The listing builds one solid part. Answer for the finished solid, in the listing's coordinates (mm). A direction names the side the tool comes from. Give positions to 0.01 mm unless a question says otherwise; leave off trailing zeros. Write each loop counter-clockwise with the first axis right and the second up, starting at its lowest first coordinate (ties: lowest second). Pieces come first, ordered by that corner, then holes.
```python
from build123d import *

# Parameters (mm, degrees)
SKETCH_1_R               = 30.6
EXTRUDE_1_DEPTH          = 24
SKETCH_3_R               = 30.6
EXTRUDE_2_DEPTH          = 0.9
EXTRUDE_2_TAPER          = 73
SKETCH_4_R               = 25.656232643
EXTRUDE_3_DEPTH          = 0.6
SKETCH_5_W               = 51
SKETCH_5_H               = 12
CUT_EXTRUDE_1_DEPTH      = 31.6000001
CUT_EXTRUDE_1_DEPTH_BACK = 31.6000001
SKETCH_6_R               = 2.65
EXTRUDE_4_DEPTH          = 13


with BuildPart() as part:
    # 草图1 → 凸台-拉伸1 (new body)
    with BuildSketch(Plane(origin=(0, 0, 0), x_dir=(1, 0, 0), z_dir=(0, 1, 0))):
        Circle(SKETCH_1_R)
    extrude(amount=EXTRUDE_1_DEPTH)

    # 草图3 → 凸台-拉伸2 (add)
    with BuildSketch(Plane(origin=(0, 24, 0), x_dir=(1, 0, 0), z_dir=(0, 1, 0))):
        Circle(SKETCH_3_R)
    extrude(amount=EXTRUDE_2_DEPTH, taper=EXTRUDE_2_TAPER)

    # 草图4 → 凸台-拉伸3 (add)
    with BuildSketch(Plane(origin=(0, 24.9, 0), x_dir=(1, 0, 0), z_dir=(0, 1, 0))):
        Circle(SKETCH_4_R)
    extrude(amount=EXTRUDE_3_DEPTH)

    # 草图5 → 切除-拉伸1 (cut, two sides)
    with BuildSketch(Plane(origin=(0, 0, 0), x_dir=(0, 0, -1), z_dir=(1, 0, 0))) as cut_extrude_1_sk:
        with Locations((0, 16)):
            Rectangle(SKETCH_5_W, SKETCH_5_H)
    extrude(amount=CUT_EXTRUDE_1_DEPTH, mode=Mode.SUBTRACT)
    extrude(cut_extrude_1_sk.sketch, amount=-CUT_EXTRUDE_1_DEPTH_BACK, mode=Mode.SUBTRACT)

    # 草图6 → 凸台-拉伸4 (add)
    with BuildSketch(Plane.XY.offset(27)):
        with Locations((0, 13)):
            Circle(SKETCH_6_R)
    extrude(amount=EXTRUDE_4_DEPTH)


solid = part.part
```
Item 1: A cutting plane is placed at B-B, the plane x = 0. Give the vertices of the cut face in (y, z), plus the area to 3 significant figures.
Conclusion:
outline: (0, -30.6) - (24, -30.6) - (24.9, -27.66) - (24.9, -25.66) - (25.5, -25.66) - (25.5, 25.66) - (24.9, 25.66) - (24.9, 27.66) - (24, 30.6) - (15.65, 30.6) - (15.65, 40) - (10.35, 40) - (10.35, 30.6) - (0, 30.6) - close; hole (10, -25.5) - (22, -25.5) - (22, 25.5) - (10, 25.5) - close
area: 990 mm2
Item 2: A cutting plane is placed at C-C, the plane y = 17.75. Give the vertices of the cut face in (x, z), plus the area to 3 significant figures.
Conclusion:
outline: (-16.91, -25.5) arc R30.6 ccw to (16.91, -25.5) - close; (-16.91, 25.5) - (16.91, 25.5) arc R30.6 ccw to start
area: 234 mm2
Item 3: Each of these flat-tipped pins is pushed along its axis until it touches: P1, Ø3, axis at x = 10.5, y = 11, coming from the -Z side; P2, Ø8, axis at y = 4.5, z = 9, coming from the -X side; P3, Ø9.5, axis at x = 2, y = 19, coming from the +Z side; P4, Ø13, axis at x = -8, y = 17.5, coming from the -Z side. Where does it stop, or does it pass through?
Conclusion:
P1: stops at z = -29.25
P2: stops at x = -30.19
P3: stops at z = 40
P4: stops at z = -30.56
Item 4: Determine the mould class of faces 4 (the face through (-3.34, 25.196, -25.438)), 5 (the face through (18.3, 24.9, 18.3)), 6 (the face through (0, 16, -25.5)) for opening direction Y: pulls with the +Y half, pulls with the -Y half, needs draft (parallel to the pull), parting line crosses it, or undercut.
Conclusion:
face 4: needs draft
face 5: pulls with the +Y half
face 6: undercut
Item 5: A cutting plane is placed at A-A, the plane y = 13. Give the vertices of the cut face in (x, z).
Conclusion:
outline: (-16.91, -25.5) arc R30.6 ccw to (16.91, -25.5) - close; (-16.91, 25.5) - (16.91, 25.5) arc R30.6 ccw to (2.65, 30.49) - (2.65, 40) - (-2.65, 40) - (-2.65, 30.49) arc R30.6 ccw to start
Item 6: A cutting plane is placed at D-D, the plane z = 31.5. Give the vertices of the cut face in (x, y).
Conclusion:
outline: circle Ø5.3 at (0, 13)
Item 7: Which of the six approach directions +Z, -Z, +X, -X, +Y, -Y give full straight-line access (tool end or side, diameter ignored) to faces 1 (the face through (0, 16, 25.5)), 2 (the face through (1.223, 10.649, 35.176)), 3 (the face through (0, 13, 40))?
Conclusion:
face 1: +X, -X
face 2: +Z
face 3: +Z, +X, -X, +Y, -Y
Item 8: Consider probe 1 along Y at (x, z) = (4, 14); probe 2 along Z at (x, y) = (-16, 20.5); probe 3 along Z at (x, y) = (13, 17). Determine where each line is inside the solid, lowest interval first.
Conclusion:
probe 1: y = 0 to 10, 22 to 25.5
probe 2: z = -26.08 to -25.5, 25.5 to 26.08
probe 3: z = -27.7 to -25.5, 25.5 to 27.7
